from build123d import *

# Parameters (mm, degrees)
F0_W        = 62.7580881119
F0_H        = 45.6833392382
F1_DEPTH    = 50
F2_T        = -2.5
F3_R        = 5
F4_T1_DEPTH = 40.6833392382
F4_T3_DEPTH = 57.7580881119
F4_T5_DEPTH = 57.7580881119


# Not quite as in the source:
# - a fillet or chamfer that OpenCascade refuses, or shapes differently, is made with other operations: its cross-section is extruded or revolved along the edge and cut away or added


with BuildPart() as f1:
    # F0 (on Front) → F1 (new body)
    with BuildSketch(Plane.XZ):
        with Locations((31.3790440559, 22.8416696191)):
            Rectangle(F0_W, F0_H)
    extrude(amount=-F1_DEPTH)

    # F2
    f2_openings = [f1.faces().sort_by_distance(p)[0] for p in [
        (31.379044, 0, 22.84167),
    ]]
    offset(amount=F2_T, openings=f2_openings)

    # F3
    f3_edges = [f1.edges().sort_by_distance(p)[0] for p in [
        (0, 25, 45.683339),
        (62.758088, 25, 45.683339),
        (62.758088, 25, 0),
        (0, 25, 0),
    ]]
    fillet(f3_edges, radius=F3_R)

    # F4: fillet of radius 5 on 5 edges, made by hand

    # F4_s2 → F4_t1 (join)
    with BuildSketch(Plane.XY.offset(2.5)):
        with BuildLine():
            ThreePointArc((2.5, 42.5), (3.9644660941, 46.0355339059), (7.5, 47.5))
            Line((7.5, 47.5), (2.5, 47.5))
            Line((2.5, 47.5), (2.5, 42.5))
        make_face()
        with BuildLine():
            ThreePointArc((60.2580881119, 42.5), (58.7936220178, 46.0355339059), (55.2580881119, 47.5))
            Line((55.2580881119, 47.5), (60.2580881119, 47.5))
            Line((60.2580881119, 47.5), (60.2580881119, 42.5))
        make_face()
    extrude(amount=F4_T1_DEPTH)

    # F4_s4 → F4_t3 (join)
    with BuildSketch(Plane.YZ.offset(2.5)):
        with BuildLine():
            ThreePointArc((42.5, 2.5), (46.0355339059, 3.9644660941), (47.5, 7.5))
            Line((47.5, 7.5), (47.5, 2.5))
            Line((47.5, 2.5), (42.5, 2.5))
        make_face()
        with BuildLine():
            ThreePointArc((42.5, 43.1833392382), (46.0355339059, 41.7188731441), (47.5, 38.1833392382))
            Line((47.5, 38.1833392382), (47.5, 43.1833392382))
            Line((47.5, 43.1833392382), (42.5, 43.1833392382))
        make_face()
    extrude(amount=F4_T3_DEPTH)

    # F4_s6 → F4_t5 (cut)
    with BuildSketch(Plane.YZ.offset(2.5)):
        with BuildLine():
            ThreePointArc((0, 48.1833392382), (1.4644660941, 44.6478053322), (5, 43.1833392382))
            Line((5, 43.1833392382), (0, 43.1833392382))
            Line((0, 43.1833392382), (0, 48.1833392382))
        make_face()
    extrude(amount=F4_T5_DEPTH, mode=Mode.SUBTRACT)


solid = f1.part
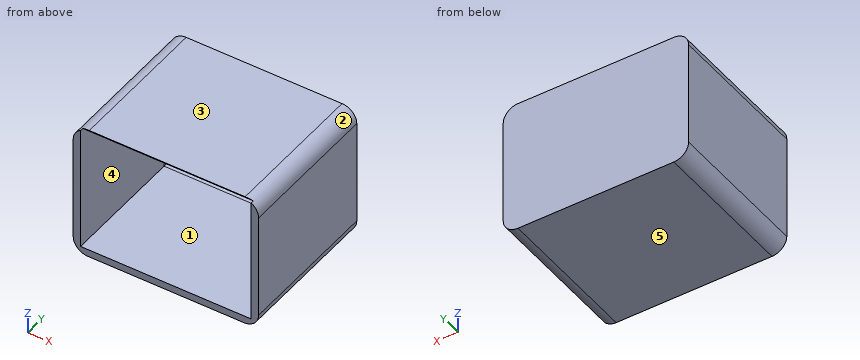
The model under review builds one solid part; all positions refer to its coordinate system, in mm. Face numbers are marked on the shaded views. A direction names the side the tool comes from. Give positions to 0.01 mm unless a question says otherwise; leave off trailing zeros. Order: outer loops, then holes, each group sorted by start corner. A loop starts at its lowest first (then second) coordinate and runs counter-clockwise, first axis right, second up. Notation, with made-up numbers: M -31,30.5 L 26,30.5 A26 cw 26,65.5 Z; hole C 87,85.25 d4. An arc over 180 degrees is marked long. Answer in a Markdown table with one row per item. Add a question column.
1. Add section A-A on y = 24. State the section outline as (x, z) points, plus the area to 3 significant figures.
2. For pin 1 Ø15.5 at (x, z) = (39.5, 21) entering from -Y, flat-tipped, find the tip position at first contact; note if it passes through.
3. Machinability: for the marked faces 1 and 2, which of the approach directions +Z, -Z, +X, -X, +Y, -Y give a long, thin tool a straight path to every point of the face, cutting with its end or side? Answer none if there is none.
4. Add section D-D on y = 46. State the section outline as (x, z) points.
5. Add section B-B on x = 37.5. State the section outline as (y, z) points.
6. To check wall thickness, follow line 1 along Z through (x, y) = (8, 20.5); line 2 along X through (y, z) = (4, 36.5); line 3 along X through (y, z) = (20.5, 41). State the ranges of each line that lie inside material, in increasing order.
7. Add section C-C on z = 27.5. State the section outline as (x, y) points, plus the area to 3 significant figures.
8. Mouldability with a two-part tool opening along Z and no side actions: class the marked faces 3, 4 and 5 as released by +Z, released by -Z, zero draft, split by the parting line, or undercut.
The answers:
| question | item | result |
|---|---|---|
| 1 | outline | M 0,5 A5 ccw 5,0 L 57.76,0 A5 ccw 62.76,5 L 62.76,40.68 A5 ccw 57.76,45.68 L 5,45.68 A5 ccw 0,40.68 Z; hole M 2.5,2.5 L 60.26,2.5 L 60.26,43.18 L 2.5,43.18 Z |
| 1 | area | 496 mm2 |
| 2 | pin 1 | y = 47.5 |
| 3 | face 1 | -Y |
| 3 | face 2 | +Z, +X, +Y, -Y |
| 4 | outline | M 0,5 A5 ccw 5,0 L 57.76,0 A5 ccw 62.76,5 L 62.76,40.68 A5 ccw 57.76,45.68 L 5,45.68 A5 ccw 0,40.68 Z; hole M 3.93,3.93 L 58.83,3.93 L 58.83,41.75 L 3.93,41.75 Z |
| 5 | outline | M 0,0 L 50,0 L 50,45.68 L 0.67,45.68 A5 ccw 5,43.18 L 42.5,43.18 A5 cw 47.5,38.18 L 47.5,7.5 A5 cw 42.5,2.5 L 0,2.5 Z |
| 6 | line 1 | 0 to 2.5, 43.18 to 45.68 |
| 6 | line 2 | 0 to 2.5, 60.26 to 62.76 |
| 6 | line 3 | 0.01 to 2.5, 60.26 to 62.75 |
| 7 | outline | M 0,0 L 2.5,0 L 2.5,42.5 A5 cw 7.5,47.5 L 55.26,47.5 A5 cw 60.26,42.5 L 60.26,0 L 62.76,0 L 62.76,50 L 0,50 Z |
| 7 | area | 405 mm2 |
| 8 | face 3 | released by +Z |
| 8 | face 4 | undercut |
| 8 | face 5 | released by -Z |
